```python
from build123d import *

# Parameters (mm, degrees)
BOX419_W          = 13
BOX419_H          = 10
BOX419_DEPTH      = 3
CYLINDER197_R     = 2
CYLINDER197_DEPTH = 20
CYLINDER199_R     = 2
CYLINDER199_DEPTH = 20
CYLINDER196_R     = 2
CYLINDER196_DEPTH = 20
CYLINDER198_R     = 2
CYLINDER198_DEPTH = 20
BOX365_W          = 3
BOX365_H          = 10
BOX365_DEPTH      = 13
BOX295_W          = 81
BOX295_H          = 10
BOX295_DEPTH      = 3
BOX366_W          = 25
BOX366_H          = 25
BOX366_DEPTH      = 3
CHAMFER024_SIZE   = 24.99
BOX293_W          = 54
BOX293_H          = 10
BOX293_DEPTH      = 3
CYLINDER065_R     = 1.25
CYLINDER065_DEPTH = 3
CYLINDER066_R     = 1.25
CYLINDER066_DEPTH = 3
CYLINDER067_R     = 1.25
CYLINDER067_DEPTH = 3
CYLINDER064_R     = 1.25
CYLINDER064_DEPTH = 3
BOX260_W          = 56
BOX260_H          = 88
BOX260_DEPTH      = 3


with BuildPart() as box419:
    # Box419 → Box419 (new body)
    with BuildSketch(Plane(origin=(-133, 66, 62), x_dir=(1, 0, 0), z_dir=(0, 0, 1))):
        with Locations((6.5, 5)):
            Rectangle(BOX419_W, BOX419_H)
    extrude(amount=BOX419_DEPTH)


with BuildPart() as cylinder197:
    # Cylinder197 → Cylinder197 (new body)
    with BuildSketch(Plane(origin=(-101, 71, 32), x_dir=(1, 0, 0), z_dir=(0, 0, 1))):
        Circle(CYLINDER197_R)
    extrude(amount=CYLINDER197_DEPTH)


with BuildPart() as cylinder199:
    # Cylinder199 → Cylinder199 (new body)
    with BuildSketch(Plane(origin=(-101, -27, 32), x_dir=(1, 0, 0), z_dir=(0, 0, 1))):
        Circle(CYLINDER199_R)
    extrude(amount=CYLINDER199_DEPTH)


with BuildPart() as cylinder196:
    # Cylinder196 → Cylinder196 (new body)
    with BuildSketch(Plane(origin=(-57, -27, 32), x_dir=(1, 0, 0), z_dir=(0, 0, 1))):
        Circle(CYLINDER196_R)
    extrude(amount=CYLINDER196_DEPTH)


with BuildPart() as fusion196:
    # Cylinder198 → Cylinder198 (new body)
    with BuildSketch(Plane(origin=(-57, 71, 32), x_dir=(1, 0, 0), z_dir=(0, 0, 1))):
        Circle(CYLINDER198_R)
    extrude(amount=CYLINDER198_DEPTH)

    # Fusion196: union Cylinder197, Cylinder199, Cylinder196
    add(cylinder197.part)
    add(cylinder199.part)
    add(cylinder196.part)


with BuildPart() as box365:
    # Box365 → Box365 (new body)
    with BuildSketch(Plane(origin=(-133, 66, 49), x_dir=(1, 0, 0), z_dir=(0, 0, 1))):
        with Locations((1.5, 5)):
            Rectangle(BOX365_W, BOX365_H)
    extrude(amount=BOX365_DEPTH)


with BuildPart() as box295:
    # Box295 → Box295 (new body)
    with BuildSketch(Plane(origin=(-133, 66, 49), x_dir=(1, 0, 0), z_dir=(0, 0, 1))):
        with Locations((40.5, 5)):
            Rectangle(BOX295_W, BOX295_H)
    extrude(amount=BOX295_DEPTH)


with BuildPart() as chamfer024:
    # Box366 → Box366 (new body)
    with BuildSketch(Plane(origin=(-133, 41, 49), x_dir=(1, 0, 0), z_dir=(0, 0, 1))):
        with Locations((12.5, 12.5)):
            Rectangle(BOX366_W, BOX366_H)
    extrude(amount=BOX366_DEPTH)

    # Chamfer024
    chamfer024_edges = [chamfer024.edges().sort_by_distance(p)[0] for p in [
        (-133, 41, 50.5),
    ]]
    chamfer(chamfer024_edges, length=CHAMFER024_SIZE)


with BuildPart() as box293:
    # Box293 → Box293 (new body)
    with BuildSketch(Plane(origin=(-106, -32, 49), x_dir=(1, 0, 0), z_dir=(0, 0, 1))):
        with Locations((27, 5)):
            Rectangle(BOX293_W, BOX293_H)
    extrude(amount=BOX293_DEPTH)


with BuildPart() as cylinder065:
    # Cylinder065 → Cylinder065 (new body)
    with BuildSketch(Plane(origin=(-51.5, 62.5, 37), x_dir=(1, 0, 0), z_dir=(0, 0, 1))):
        Circle(CYLINDER065_R)
    extrude(amount=CYLINDER065_DEPTH)


with BuildPart() as cylinder066:
    # Cylinder066 → Cylinder066 (new body)
    with BuildSketch(Plane(origin=(-51.5, 4.5, 37), x_dir=(1, 0, 0), z_dir=(0, 0, 1))):
        Circle(CYLINDER066_R)
    extrude(amount=CYLINDER066_DEPTH)


with BuildPart() as cylinder067:
    # Cylinder067 → Cylinder067 (new body)
    with BuildSketch(Plane(origin=(-100.5, 4.5, 37), x_dir=(1, 0, 0), z_dir=(0, 0, 1))):
        Circle(CYLINDER067_R)
    extrude(amount=CYLINDER067_DEPTH)


with BuildPart() as fusion193:
    # Cylinder064 → Cylinder064 (new body)
    with BuildSketch(Plane(origin=(-100.5, 62.5, 37), x_dir=(1, 0, 0), z_dir=(0, 0, 1))):
        Circle(CYLINDER064_R)
    extrude(amount=CYLINDER064_DEPTH)

    # Fusion193: union Cylinder065, Cylinder066, Cylinder067
    add(cylinder065.part)
    add(cylinder066.part)
    add(cylinder067.part)


with BuildPart() as fusion262:
    # Box260 → Box260 (new body)
    with BuildSketch(Plane(origin=(-104, -22, 37), x_dir=(1, 0, 0), z_dir=(0, 0, 1))):
        with Locations((28, 44)):
            Rectangle(BOX260_W, BOX260_H)
    extrude(amount=BOX260_DEPTH)

    # Cut251: cut Fusion193
    add(fusion193.part, mode=Mode.SUBTRACT)


with BuildPart() as fusion262_1:
    # Cut251 placement: moved
    add(fusion262.part.moved(Location((-4, 0, 12))))

    # Fusion194: union Box295, Chamfer024, Box293
    add(box295.part)
    add(chamfer024.part)
    add(box293.part)

    # Fusion195: union Box365
    add(box365.part)

    # Cut252: cut Fusion196
    add(fusion196.part, mode=Mode.SUBTRACT)

    # Fusion262: union Box419
    add(box419.part)


solid = fusion262_1.part
```
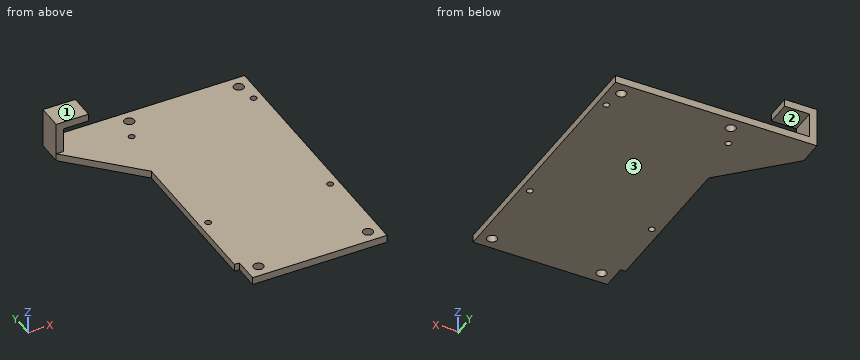
The listing builds one solid part. Answer for the finished solid, in the listing's coordinates (mm). Face numbers are marked on the shaded views. Give positions to 0.01 mm unless a question says otherwise; leave off trailing zeros. Order: outer loops, then holes, each group sorted by start corner. A loop starts at its lowest first (then second) coordinate and runs counter-clockwise, first axis right, second up. Notation, with made-up numbers: M 87.25,-23 L 127.25,-23 A23 cw 127.25,12 Z; hole C -7,33 d2. An arc over 180 degrees is marked long. Put each result on its own line as item: value. Start each with the question number.
Item 1: The part is cut by section A-A, the plane y = 62.5. Determine the outline of the cut face in (x, z).
Item 2: Flat-ended cylindrical pins translate along their axes: P1, Ø3, axis at x = -101, y = 71, coming from the +Z side; P2, Ø2.5, axis at y = 14, z = 50, coming from the -X side; P3, Ø0.9, axis at y = -28.5, z = 50, coming from the -X side; P4, Ø12, axis at x = -79, y = 18, coming from the +Z side. Find the tip coordinate at first contact, or state that the pin passes through.
Item 3: The part is cut by section D-D, the plane x = -118.5. Determine the outline of the cut face in (y, z).
Item 4: The part is cut by section C-C, the plane y = 44. Determine the outline of the cut face in (x, z).
Item 5: The part is cut by section B-B, the plane x = -104.5. Determine the outline of the cut face in (y, z).
Item 6: For a pull along Z with two mould halves and no side action, classify the marked faces 1, 2 and 3 as +Z half, -Z half, draft (parallel to the pull), parting line (faces both ways), or undercut.
Item 7: Find the intervals of material crossed by line 1 along Y through (x, z) = (-104.5, 50.9); line 2 along X through (y, z) = (71, 50.1); line 3 along Y through (x, z) = (-101, 50.65), in increasing order.
Answer key:
1. outline: M -129.51,49 L -105.75,49 L -105.75,52 L -129.51,52 Z; M -103.25,49 L -56.75,49 L -56.75,52 L -103.25,52 Z; M -54.25,49 L -52,49 L -52,52 L -54.25,52 Z
2. P1: passes through
2. P2: stops at x = -108
2. P3: stops at x = -106
2. P4: stops at z = 52
3. outline: M 51.49,49 L 76,49 L 76,52 L 51.49,52 Z
4. outline: M -111.01,49 L -52,49 L -52,52 L -111.01,52 Z
5. outline: M -32,49 L 3.25,49 L 3.25,52 L -32,52 Z; M 5.75,49 L 61.25,49 L 61.25,52 L 5.75,52 Z; M 63.75,49 L 76,49 L 76,52 L 63.75,52 Z
6. face 1: +Z half
6. face 2: undercut
6. face 3: -Z half
7. line 1: y = -32 to 3.25, 5.75 to 61.25, 63.75 to 76
7. line 2: x = -133 to -103, -99 to -59, -55 to -52
7. line 3: y = -32 to -29, -25 to 69, 73 to 76
